Autodesk Inventor part; units mm, degrees
ref_plane "YZ Plane" through (0, 0, 0) normal (1, 0, 0) x (0, 1, 0)
ref_plane "XZ Plane" through (0, 0, 0) normal (0, 1, 0) x (-1, 0, 0)
ref_plane "XY Plane" through (0, 0, 0) normal (0, 0, 1) x (1, 0, 0)
sketch "Sketch1" plane through (0, 0, 0) normal (0, 1, 0) x (-1, 0, 0)
  line L0 (12, 0) -> (12, 0)
  line L1 (24, -12) -> (24, -34)
  line L2 (0, -34) -> (0, -12)
  arc A0 (24, -12) -> (12, 0) centre (12, -12) ccw
  arc A1 (12, 0) -> (0, -12) centre (12, -12) ccw
  line L3 (0, -34) -> (-29, -34)
  line L4 (-29, -34) -> (-29, -62)
  line L5 (-29, -62) -> (-20, -62)
  line L6 (-20, -62) -> (-20, -42)
  line L7 (-20, -42) -> (21, -42)
  line L8 (21, -42) -> (21, -62)
  line L9 (21, -62) -> (30, -62)
  line L10 (30, -62) -> (30, -34)
  line L11 (30, -34) -> (24, -34)
  line L12 (25.5, -62) -> (25.5, -57)
  line L13 (25.5, -57) -> (25.5, -47)
  circle A2 centre (25.5, -57) radius 1.5
  circle A3 centre (25.5, -47) radius 1.5
  line L14 (25.5, -57) -> (-24.5, -57)
  line L15 (-24.5, -57) -> (-24.5, -47)
  circle A4 centre (-24.5, -47) radius 1.5
  circle A5 centre (-24.5, -57) radius 1.5
  point P0 (0, 0)
  point P1 (24, 0)
  dimension "d0" = 24
  dimension "d1" = 34
  dimension "d2" = 12
  dimension "d3" = 29
  dimension "d4" = 28
  dimension "d5" = 9
  dimension "d6" = 20
  dimension "d7" = 41
  dimension "d8" = 9
  dimension "d9" = 5
  dimension "d10" = 10
  dimension "d11" = 3
  dimension "d12" = 3
  dimension "d13" = 3
  dimension "d14" = 3
extrude "Extrusion1" add sketch "Sketch1" along normal blind 1 contours L1 L11 L10 L9 L12 A2 L14 L8 L7 L6 L5 L4 L3 L2 A1 A0 | L9 L8 L14 A2 L12
sketch "Sketch2" plane through (0, 1, 0) normal (0, 1, 0) x (1, 0, 0)
  arc A0 (-24, 12) -> (0, 12) centre (-12, 12) ccw
  circle A1 centre (-25.5, 57) radius 1.5
  circle A2 centre (-25.5, 47) radius 1.5
  line L0 (-25.5, 57) -> (-25.5, 47)
  line L1 (-12, 12) -> (-12, 19)
  line L2 (-12, 19) -> (-12, 5)
  circle A3 centre (-12, 5) radius 1.5
  circle A4 centre (-12, 19) radius 1.5
  point P0 (0, 0)
  dimension "d17" = 7
  dimension "d18" = 14
  dimension "d19" = 3
  dimension "d20" = 3
extrude "Extrusion2" cut sketch "Sketch2" against normal blind 1 contours A4 | A3
properties part number "Wrist Servo Plate"
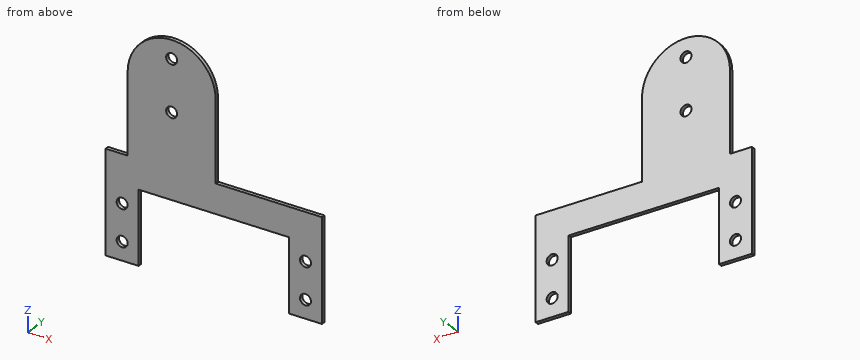
Part model, mm, in its own coordinate system. Round coordinates to 2 decimals unless told otherwise and drop trailing zeros. Order: outer loops, then holes, each group sorted by start corner. A loop starts at its lowest first (then second) coordinate and runs counter-clockwise, first axis right, second up. Notation, with made-up numbers: M 3,-20.5 L 45,-20.5 A27 ccw 45,15.5 Z; hole C 9.5,16.5 d7. An arc over 180 degrees is marked long. Put each result on its own line as item: value. Start each with the question number.
1. Slice it at B-B on x = -25.5. List the corners of the cut face in (y, z).
2. Slice it at A-A on z = -54.5. List the corners of the cut face in (x, y), then the cut area to 3 significant figures.
3. Drop flat-ended pins along their axis: pin 1 (1.8 mm diameter, centred on x = 24.5, z = -47, fed in from +Y); pin 2 (0.5 mm diameter, centred on x = 17.5, y = 0.5, fed in from +Z); pin 3 (0.5 mm diameter, centred on y = 0.5, z = -25, fed in from -X). Give the stop position or say it passes through.
4. Slice it at C-C on y = 0.15. List the corners of the cut face in (x, z).
5. Slice it at D-D on z = -19. List the corners of the cut face in (x, y), then the cut area to 3 significant figures.
6. Drill centre lines: probe 1 along Z at (x, y) = (-25.5, 0.65); probe 2 along X at (y, z) = (0.85, -57); probe 3 along Z at (x, y) = (-12, 0.5). Where is each one in solid material? Low to high. Write a range as [from, to].
Findings:
1. outline: M 0,-62 L 1,-62 L 1,-58.5 L 0,-58.5 Z; M 0,-55.5 L 1,-55.5 L 1,-48.5 L 0,-48.5 Z; M 0,-45.5 L 1,-45.5 L 1,-34 L 0,-34 Z
2. outline: M -30,0 L -21,0 L -21,1 L -30,1 Z; M 20,0 L 29,0 L 29,1 L 20,1 Z
2. area: 18.0 mm2
3. pin 1: through
3. pin 2: z = -34
3. pin 3: x = -24
4. outline: M -30,-62 L -21,-62 L -21,-42 L 20,-42 L 20,-62 L 29,-62 L 29,-34 L 0,-34 L 0,-12 A12 ccw -24,-12 L -24,-34 L -30,-34 Z; hole C -25.5,-57 d3; hole C -25.5,-47 d3; hole C -12,-19 d3; hole C -12,-5 d3; hole C 24.5,-57 d3; hole C 24.5,-47 d3
5. outline: M -24,0 L -13.5,0 L -13.5,1 L -24,1 Z; M -10.5,0 L 0,0 L 0,1 L -10.5,1 Z
5. area: 21.0 mm2
6. probe 1: [-62, -58.5], [-55.5, -48.5], [-45.5, -34]
6. probe 2: [-30, -27], [-24, -21], [20, 23], [26, 29]
6. probe 3: [-42, -20.5], [-17.5, -6.5], [-3.5, 0]
